```python
from build123d import *
from build123d.topology import SkipClean

# Parameters (mm, degrees)
BOSS_EXTRUDE1_DEPTH      = 20
BOSS_EXTRUDE1_DEPTH_BACK = 5
BOSS_EXTRUDE2_START      = -5
BOSS_EXTRUDE2_DEPTH      = 5
BOSS_EXTRUDE3_DEPTH      = 70


with BuildPart() as part:
    # Sketch1 → Boss-Extrude1 (new, two sides: drawn at the far end of the back side and taken through both)
    with BuildSketch(Plane.XY.offset(-BOSS_EXTRUDE1_DEPTH_BACK)):
        with BuildLine():
            Line((0, 25), (0, 17))
            ThreePointArc((0, 17), (-17, 0), (0, -17))
            Line((0, -17), (0, -25))
            ThreePointArc((0, -25), (-25, 0), (0, 25))
        make_face()
    extrude(amount=BOSS_EXTRUDE1_DEPTH + BOSS_EXTRUDE1_DEPTH_BACK)

    # Sketch2 → Boss-Extrude2 (add)
    with BuildSketch(Plane.XY.offset(BOSS_EXTRUDE2_START)):
        with BuildLine():
            Line((0, -25), (0, -72.5))
            ThreePointArc((0, -72.5), (-61.581037686, -38.262590053), (-65, 32.113081447))
            Line((-65, 32.113081447), (-65, 77))
            Line((-65, 77), (0, 77))
            Line((0, 77), (0, 25))
            Line((0, 25), (0, 17))
            ThreePointArc((0, 17), (-17, 0), (0, -17))
            Line((0, -17), (0, -25))
        make_face()
    extrude(amount=BOSS_EXTRUDE2_DEPTH)


with BuildPart() as body_2:
    # Mirror8: mirrored copy
    add(part.part.mirror(Plane.XY.offset(-40)))


with BuildPart() as part_1:
    add(part.part)

    add(body_2.part)  # Boss-Extrude3 merges body 2
    # Sketch3 → Boss-Extrude3 (add)
    with BuildSketch(Plane.XY.offset(-75)):
        with BuildLine():
            Line((-65, 32.113081447), (-65, 77))
            Line((-65, 77), (-60, 77))
            Line((-60, 77), (-60, 32.113081447))
            ThreePointArc((-60, 32.113081447), (-58.380864924, -34.970339014), (0, -68.053287944))
            Line((0, -68.053287944), (0, -72.5))
            ThreePointArc((0, -72.5), (-61.581037686, -38.262590053), (-65, 32.113081447))
        make_face()
    extrude(amount=BOSS_EXTRUDE3_DEPTH)

    # Mirror9: part across plane


with BuildPart() as part_2:
    with SkipClean():  # the faces are left unmerged after this step: merging them gives an invalid solid
        add(part_1.part)
        add(part_1.part.mirror(Plane(origin=(0, 0, 0), x_dir=(0, 0, 1), z_dir=(1, 0, 0))))


solid = part_2.part
```
Work out the finished part from the listing and answer in its coordinate system (mm). A direction names the side the tool comes from. Give positions to 0.01 mm unless a question says otherwise; leave off trailing zeros. Write each loop counter-clockwise with the first axis right and the second up, starting at its lowest first coordinate (ties: lowest second). Pieces come first, ordered by that corner, then holes. Notation, with made-up numbers: (-9, 20.5) -> (2, 20.5) arc R17 ccw to (2, 53.5) -> close; hole circle Ø6 at (-14, 45). An arc over 180 degrees is marked (long way). Write each question's results on one line, items separated by ' | '.
1. Find section C-C on z = -44. Determine the outline of the cut face in (x, y).
Data:
outline: (-65, 32.11) arc R72.5 ccw (long way) to (65, 32.11) -> (65, 77) -> (60, 77) -> (60, 32.11) arc R68.05 cw (long way) to (-60, 32.11) -> (-60, 77) -> (-65, 77) -> close
2. A tool of negligible diameter and unlimited length cuts with its end or side. For faces 4 (the flat face through (-17, 20, -80)), 5 (the flat face through (65, 54, -41)), 6 (the flat face through (60, 55, -40)), from which of +Z, -Z, +X, -X, +Y, -Y can it reach the whole face along a straight path? Write none if from no direction.
Data:
face 4: -Z | face 5: +Z, -Z, +X, +Y | face 6: +Y
3. Find section A-A on y = 0. Determine the outline of the cut face in (x, z), and give its area (3 significant figures).
Data:
outline: (-72.5, -80) -> (-25, -80) -> (-25, -100) -> (-17, -100) -> (-17, -75) -> (-68.05, -75) -> (-68.05, -5) -> (-17, -5) -> (-17, 20) -> (-25, 20) -> (-25, 0) -> (-72.5, 0) -> close; (17, -100) -> (25, -100) -> (25, -80) -> (72.5, -80) -> (72.5, 0) -> (25, 0) -> (25, 20) -> (17, 20) -> (17, -5) -> (68.05, -5) -> (68.05, -75) -> (17, -75) -> close | area: 2,370 mm^2
4. Each of these flat-tipped pins is pushed along its axis until it touches: pin 1 Ø3 at (x, z) = (57.5, -31) entering from +Y; pin 2 Ø12 at (x, y) = (-57, 30) entering from +Z; pin 3 Ø1.5 at (y, z) = (4, -32.5) entering from -X. Where does it stop, or does it pass through?
Data:
pin 1: y = -33.92 | pin 2: z = 0 | pin 3: x = -72.43
5. Determine the mould class of faces 1 (the flat face through (-65, 54, -41)), 2 (the flat face through (-17, 20, 0)), 3 (the flat face through (-60, 55, -40)) for opening direction X: +X half, -X half, draft (parallel to the pull), parting line (faces both ways), or undercut.
Data:
face 1: -X half | face 2: draft | face 3: undercut
6. Straight lines are drawn through the part: L1, parallel to Z at x = -12, y = 31.5; L2, parallel to Z at x = 5, y = 24; L3, parallel to X at y = -1, z = -20. For each, find the intervals that lie inside material, in ascending order.
Data:
L1: -80 to -75, -5 to 0 | L2: -100 to -75, -5 to 20 | L3: -72.49 to -68.05, 68.05 to 72.49
7. Find section D-D on y = 47.5. Determine the outline of the cut face in (x, z).
Data:
outline: (-65, -80) -> (65, -80) -> (65, 0) -> (-65, 0) -> close; hole (-60, -75) -> (60, -75) -> (60, -5) -> (-60, -5) -> close
8. Find section B-B on x = -10. Determine the outline of the cut face in (y, z), and give its area (3 significant figures).
Data:
outline: (-71.81, -80) -> (-22.91, -80) -> (-22.91, -100) -> (-13.75, -100) -> (-13.75, -75) -> (-67.31, -75) -> (-67.31, -5) -> (-13.75, -5) -> (-13.75, 20) -> (-22.91, 20) -> (-22.91, 0) -> (-71.81, 0) -> close; (13.75, -100) -> (22.91, -100) -> (22.91, -80) -> (77, -80) -> (77, -75) -> (13.75, -75) -> close; (13.75, -5) -> (77, -5) -> (77, 0) -> (22.91, 0) -> (22.91, 20) -> (13.75, 20) -> close | area: 2,260 mm^2
